Input: part model. Units: mm. Frame: model coordinates. A direction names the side the tool comes from. Give positions to 0.01 mm unless a question says otherwise; leave off trailing zeros. Loops run counter-clockwise (first coordinate to the right, second up) from the corner with the lowest first, then second, coordinate; pieces in that order, holes last. Notation, with made-up numbers: (37, 52.25) -> (69, 52.25) arc R28 ccw to (69, 90.25) -> close; hole circle Ø5 at (-1.75, -1.75). An arc over 180 degrees is marked (long way). Use CSV: the item, a comma, the result in double quotes.
```python
from build123d import *

# Parameters (mm, degrees)
CROQUIS1_R              = 1.6
SALIENTE_EXTRUIR1_DEPTH = 2.5
CROQUIS3_R              = 1.5
CORTAR_EXTRUIR1_DEPTH   = 5
CORTAR_EXTRUIR2_DEPTH   = 25


with BuildPart() as part:
    # Croquis1 → Saliente-Extruir1 (new, symmetric)
    with BuildSketch(Plane.XY):
        with BuildLine():
            Line((-22, -17.5), (22, -17.5))
            ThreePointArc((22, -17.5), (24.121320344, -16.621320344), (25, -14.5))
            Line((25, -14.5), (25, 14.5))
            ThreePointArc((25, 14.5), (24.121320344, 16.621320344), (22, 17.5))
            Line((22, 17.5), (-22, 17.5))
            ThreePointArc((-22, 17.5), (-24.121320344, 16.621320344), (-25, 14.5))
            Line((-25, 14.5), (-25, -14.5))
            ThreePointArc((-25, -14.5), (-24.121320344, -16.621320344), (-22, -17.5))
        make_face()
        with Locations((-19.4, 12.9)):
            Circle(CROQUIS1_R, mode=Mode.SUBTRACT)
        with Locations(Location((19.4, 12.9, 0), (0, 0, 180))):
            Circle(CROQUIS1_R, mode=Mode.SUBTRACT)
        with Locations((19.4, -12.9)):
            Circle(CROQUIS1_R, mode=Mode.SUBTRACT)
        with Locations(Location((-19.4, -12.9, 0), (0, 0, 180))):
            Circle(CROQUIS1_R, mode=Mode.SUBTRACT)
    extrude(amount=SALIENTE_EXTRUIR1_DEPTH, both=True)

    # Croquis2 → Revolución1 (revolve)
    with BuildSketch(Plane(origin=(0, 0, 0), x_dir=(1, 0, 0), z_dir=(0, 1, 0))):
        Polygon((8.2, 2.5), (8.2, 12.5), (14.7, 12.5), (14.7, 5.5), (17, 2.5), align=None)
    revolve(axis=Axis((0, 0, 7.417580073), (0, 0, -1)))

    # Croquis3 → Cortar-Extruir1 (cut)
    with BuildSketch(Plane(origin=(0, 0, -2.5), x_dir=(-1, 0, 0), z_dir=(0, 0, -1))):
        Circle(CROQUIS3_R)
    extrude(amount=-CORTAR_EXTRUIR1_DEPTH, mode=Mode.SUBTRACT)

    # Croquis4 → Cortar-Extruir2 (cut)
    with BuildSketch(Plane.XY.offset(2.5)):
        with BuildLine():
            Line((-10, 17.5), (10, 17.5))
            ThreePointArc((10, 17.5), (0, 14.466629547), (-10, 17.5))
        make_face()
    extrude(amount=-CORTAR_EXTRUIR2_DEPTH, mode=Mode.SUBTRACT)


solid = part.part
```
1) Ray query, line 1 (Y direction, x = 19.4, z = 0.8); line 2 (X direction, y = 0, z = -8); line 3 (Z direction, x = -20, y = -3.5). Return the intervals inside material, ascending.
From the geometry:
line 1,"y = -17.5 to -14.5, -11.3 to 11.3, 14.5 to 17.5"
line 2,"x = -14.7 to -8.2, 8.2 to 14.7"
line 3,"z = -2.5 to 2.5"
2) Reachability of faces 1 (the flat face through (25, 0, 0)), 2 (the flat face through (0, -2, -2.5)) from +Z, -Z, +X, -X, +Y, -Y: full face, straight path, thin tool, end or side. Return the list, or none.
From the geometry:
face 1,"+Z, -Z, +X, +Y, -Y"
face 2,"-Z"
3) Contact query for flat-ended pins moving along their axis: pin 1 (8 mm diameter, centred on y = -6, z = -5, fed in from +X); pin 2 (3.5 mm diameter, centred on x = 19.4, y = 12.9, fed in from -Z); pin 3 (2 mm diameter, centred on x = 5.5, z = -2, fed in from +Y); pin 4 (5 mm diameter, centred on x = 15, z = -11, fed in from +Y). Output: stop coordinate, or through.
From the geometry:
pin 1,"stops at x = 25"
pin 2,"stops at z = -2.5"
pin 3,"stops at y = 15.68"
pin 4,"stops at y = 7.74"
4) Section query A-A (x = 0). Return loops of the section in (y, z).
From the geometry:
outline,"(-17.5, -2.5) -> (-17, -2.5) -> (-14.7, -5.5) -> (-14.7, -12.5) -> (-8.2, -12.5) -> (-8.2, -2.5) -> (-1.5, -2.5) -> (-1.5, 2.5) -> (-17.5, 2.5) -> close; (1.5, -2.5) -> (8.2, -2.5) -> (8.2, -12.5) -> (14.47, -12.5) -> (14.47, 2.5) -> (1.5, 2.5) -> close"
5) Mould query, pull axis X, two halves, no side actions, for faces 3 (the cylindrical face through (24.1, -16.64, 0.04)), 4 (the flat face through (-16, 17.5, 0)), 5 (the cylindrical face through (-1.07, -8.13, -7.57)). Classes: pulls with the +X half, pulls with the -X half, needs draft (parallel to the pull), parting line crosses it, or undercut.
From the geometry:
face 3,"pulls with the +X half"
face 4,"needs draft"
face 5,"undercut"
6) Section query B-B (z = 1). Return loops of the section in (x, y).
From the geometry:
outline,"(-25, -14.5) arc R3 ccw to (-22, -17.5) -> (22, -17.5) arc R3 ccw to (25, -14.5) -> (25, 14.5) arc R3 ccw to (22, 17.5) -> (10, 17.5) arc R18 cw to (-10, 17.5) -> (-22, 17.5) arc R3 ccw to (-25, 14.5) -> close; hole circle Ø3.2 at (-19.4, -12.9); hole circle Ø3.2 at (-19.4, 12.9); hole circle Ø3 at (0, 0); hole circle Ø3.2 at (19.4, -12.9); hole circle Ø3.2 at (19.4, 12.9)"
7) Section query C-C (x = -19.4). Return loops of the section in (y, z).
From the geometry:
outline,"(-17.5, -2.5) -> (-14.5, -2.5) -> (-14.5, 2.5) -> (-17.5, 2.5) -> close; (-11.3, -2.5) -> (11.3, -2.5) -> (11.3, 2.5) -> (-11.3, 2.5) -> close; (14.5, -2.5) -> (17.5, -2.5) -> (17.5, 2.5) -> (14.5, 2.5) -> close"
8) Section query D-D (y = 0). Return loops of the section in (x, z).
From the geometry:
outline,"(-25, -2.5) -> (-17, -2.5) -> (-14.7, -5.5) -> (-14.7, -12.5) -> (-8.2, -12.5) -> (-8.2, -2.5) -> (-1.5, -2.5) -> (-1.5, 2.5) -> (-25, 2.5) -> close; (1.5, -2.5) -> (8.2, -2.5) -> (8.2, -12.5) -> (14.7, -12.5) -> (14.7, -5.5) -> (17, -2.5) -> (25, -2.5) -> (25, 2.5) -> (1.5, 2.5) -> close"
